Autodesk Inventor part; units mm, degrees
ref_plane "YZ Plane" through (0, 0, 0) normal (1, 0, 0) x (0, 1, 0)
ref_plane "XZ Plane" through (0, 0, 0) normal (0, 1, 0) x (-1, 0, 0)
ref_plane "XY Plane" through (0, 0, 0) normal (0, 0, 1) x (1, 0, 0)
sketch "Sketch5" plane through (0, 0, 0) normal (0, 1, 0) x (-1, 0, 0)
  arc A0 (0, -50.8) -> (0, 50.8) centre (0, 0) ccw
  line L0 (0, -50.8) -> (-38.1, -50.8)
  line L1 (0, 50.8) -> (-38.1, 50.8)
  line L2 (-38.1, 50.8) -> (-38.1, -50.8)
  dimension "d13" = 101.6
  dimension "d14" = 38.1
  dimension "d15" = 38.1
extrude "Extrusion2" add sketch "Sketch5" along normal blind 19.05
sketch "Sketch6" plane through (0, 19.05, 0) normal (0, 1, 0) x (1, 0, 0)
  arc A0 (0, 25.4) -> (0, -25.4) centre (0, 0) ccw
  line L0 (0, 25.4) -> (38.1, 25.4)
  line L1 (38.1, -50.8) -> (38.1, 50.8)
  line L2 (0, -25.4) -> (38.1, -25.4)
  line L3 (38.1, 25.4) -> (38.1, -25.4)
  dimension "d18" = 50.8
extrude "Extrusion3" add sketch "Sketch6" along normal blind 50.8
sketch "Sketch7" plane through (0, 69.85, 0) normal (0, 1, 0) x (1, 0, 0)
  arc A0 (0, 16.51) -> (0, -16.51) centre (0, 0) ccw
  line L0 (0, 16.51) -> (38.1, 16.51)
  line L1 (38.1, -25.4) -> (38.1, 25.4)
  line L2 (0, -16.51) -> (38.1, -16.51)
  dimension "d21" = 33.02
extrude "Extrusion4" cut sketch "Sketch7" against normal blind 17.78
sketch "Sketch9" plane through (0, 0, 0) normal (0, -1, 0) x (1, 0, 0)
  arc A0 (0, 38.1) -> (0, -38.1) centre (0, 0) ccw
  circle A1 centre (-38.1, 0) radius 5.08
  circle A2 centre (0, 38.1) radius 5.08
  circle A3 centre (0, -38.1) radius 5.08
  dimension "d24" = 76.2
  dimension "d25" = 10.16
  dimension "d27" = 10.16
  dimension "d28" = 10.16
extrude "Extrusion5" cut sketch "Sketch9" against normal blind 19.05
sketch "Sketch10" plane through (0, 19.05, 0) normal (0, 1, 0) x (1, 0, 0)
  circle A0 centre (0, -38.1) radius 5.08
  circle A1 centre (0, -38.1) radius 8.89
  circle A2 centre (-38.1, 0) radius 5.08
  circle A3 centre (0, 38.1) radius 5.08
  circle A4 centre (-38.1, 0) radius 8.89
  circle A5 centre (0, 38.1) radius 8.89
  point P0 (0, 0)
  dimension "d31" = 17.78
  dimension "d35" = 17.78
extrude "Extrusion6" cut sketch "Sketch10" against normal blind 3.81
mirror "Mirror1" about plane through (38.1, 0, 50.8) normal (1, 0, 0)
properties part number "Problem14_36_JacobMorgan_030916_pd3" material "Steel, Mild"
Verification items for the finished model (mm, model axes). A direction names the side the tool comes from. Coordinates: 2 decimals unless noted, no trailing zeros. Order: outer loops, then holes, each group sorted by start corner. A loop starts at its lowest first (then second) coordinate and runs counter-clockwise, first axis right, second up. Notation, with made-up numbers: (-7, 50) -> (33, 50) arc R26 ccw to (33, 84) -> close; hole circle Ø5 at (1, 87.25). An arc over 180 degrees is marked (long way). Use CSV: the item, a comma, the result in double quotes. Start each with the question number.
Q1. Section check A-A, the plane y = 57. Record the cut outline in (x, z).
Q2. Section check C-C, the plane z = 3. Record the cut outline in (x, y).
Q3. Section check D-D, the plane x = 18. Record the cut outline in (y, z), and give its area (3 significant figures).
Q4. Section check B-B, the plane x = -2. Record the cut outline in (y, z), and give its area (3 significant figures).
Q5. Depth check by flat-ended pin: P1, Ø19.5, axis at x = 80, z = 41.5, coming from the +Y side; P2, Ø15, axis at x = 25, y = 57, coming from the -Z side; P3, Ø8, axis at y = 59, z = -3, coming from the +X side. Enter the tip coordinate at first touch or a pass-through.
Q6. Thickness scan on line 1 along Z through (x, y) = (76, 4); line 2 along X through (y, z) = (17.5, 0); line 3 along Z through (x, y) = (76, 17). Record the ranges inside material, lowest first.
Q7. Tool access check on faces 1 (the cylindrical face through (-25.394, 44.094, 0.559)), 2 (the cylindrical face through (-1.93, 17.17, -29.42)), 3 (the flat face through (38, 44, -25.4)). Record the directions out of +Z, -Z, +X, -X, +Y, -Y that give a thin tool (end or side, any length) a straight path to the whole face; none if there is none.
Returned:
1,outline,"(0, -25.4) -> (76.2, -25.4) arc R25.4 ccw to (76.2, 25.4) -> (0, 25.4) arc R25.4 ccw to start; hole (0, -16.51) -> (76.2, -16.51) arc R16.51 ccw to (76.2, 16.51) -> (0, 16.51) arc R16.51 ccw to start"
2,outline,"(-50.71, 0) -> (-42.2, 0) -> (-42.2, 15.24) -> (-46.47, 15.24) -> (-46.47, 19.05) -> (-50.71, 19.05) -> close; (-34, 0) -> (110.2, 0) -> (110.2, 15.24) -> (105.93, 15.24) -> (105.93, 19.05) -> (101.42, 19.05) -> (101.42, 69.85) -> (92.44, 69.85) -> (92.44, 52.07) -> (-16.24, 52.07) -> (-16.24, 69.85) -> (-25.22, 69.85) -> (-25.22, 19.05) -> (-29.73, 19.05) -> (-29.73, 15.24) -> (-34, 15.24) -> close; (118.4, 0) -> (126.91, 0) -> (126.91, 19.05) -> (122.67, 19.05) -> (122.67, 15.24) -> (118.4, 15.24) -> close"
3,outline,"(0, -50.8) -> (19.05, -50.8) -> (19.05, -25.4) -> (69.85, -25.4) -> (69.85, -16.51) -> (52.07, -16.51) -> (52.07, 16.51) -> (69.85, 16.51) -> (69.85, 25.4) -> (19.05, 25.4) -> (19.05, 50.8) -> (0, 50.8) -> close"
3,area,"3,930 mm^2"
4,outline,"(0, -50.76) -> (19.05, -50.76) -> (19.05, -46.76) -> (15.24, -46.76) -> (15.24, -42.77) -> (0, -42.77) -> close; (0, -33.43) -> (15.24, -33.43) -> (15.24, -29.44) -> (19.05, -29.44) -> (19.05, -25.32) -> (69.85, -25.32) -> (69.85, -16.39) -> (52.07, -16.39) -> (52.07, 16.39) -> (69.85, 16.39) -> (69.85, 25.32) -> (19.05, 25.32) -> (19.05, 29.44) -> (15.24, 29.44) -> (15.24, 33.43) -> (0, 33.43) -> close; (0, 42.77) -> (15.24, 42.77) -> (15.24, 46.76) -> (19.05, 46.76) -> (19.05, 50.76) -> (0, 50.76) -> close"
4,area,"3,510 mm^2"
5,P1,"stops at y = 19.05"
5,P2,"stops at z = -25.4"
5,P3,"stops at x = 101.6"
6,line 1,"z = -50.8 to -43.18, -33.02 to 33.02, 43.18 to 50.8"
6,line 2,"x = -50.8 to -46.99, -29.21 to 105.41, 123.19 to 127"
6,line 3,"z = -50.8 to -46.99, -29.21 to 29.21, 46.99 to 50.8"
7,face 1,"-X, +Y"
7,face 2,"+Y"
7,face 3,"-Z, +X, -X, +Y"
